```python
from build123d import *

# Parameters (mm, degrees)
F1_DEPTH = 6.35
F2_W     = 6.35
F2_H     = 55.88
F3_DEPTH = 33.64992
F4_SIZE  = 27.94
F5_R     = 10.64163
F6_DEPTH = 38.101


with BuildPart() as f1:
    # F0 (on Top) → F1 (new body)
    with BuildSketch(Plane.XY):
        Polygon((19.05, 27.94), (0, 27.94), (-19.05, 27.94), (-19.05, 0), (-19.05, -27.94), (0, -27.94), (19.05, -27.94), (19.05, 0), align=None)
    extrude(amount=F1_DEPTH)

    # F2 (on face) → F3 (join)
    with BuildSketch(Plane.XY.offset(6.35)):
        with Locations((-15.875, 0)):
            Rectangle(F2_W, F2_H)
        with Locations((15.875, 0)):
            Rectangle(F2_W, F2_H)
    extrude(amount=F3_DEPTH)

    # F4
    f4_edges = [f1.edges().sort_by_distance(p)[0] for p in [
        (15.875, -27.94, 39.99992),
        (-15.875, -27.94, 39.99992),
    ]]
    chamfer(f4_edges, length=F4_SIZE)

    # F5 (on face) → F6 (cut, through all)
    with BuildSketch(Plane.YZ.offset(19.05)):
        with Locations((13.47094, 19.69512)):
            Circle(F5_R)
    extrude(amount=-F6_DEPTH, mode=Mode.SUBTRACT)


solid = f1.part
```
Build history of the part. All positions in model axes, mm. A direction names the side the tool comes from. Give positions to 0.01 mm unless a question says otherwise; leave off trailing zeros. Loops run counter-clockwise (first coordinate to the right, second up) from the corner with the lowest first, then second, coordinate; pieces in that order, holes last.
Item 1: Slice it at B-B, the plane y = 1.5. List the corners of the cut face in (x, z), and give its area (3 significant figures).
Answers follow:
outline: (-19.05, 0) - (19.05, 0) - (19.05, 40) - (12.7, 40) - (12.7, 6.35) - (-12.7, 6.35) - (-12.7, 40) - (-19.05, 40) - close
area: 669 mm2
Item 2: Which spindle directions (+Z, -Z, +X, -X, +Y, -Y) get a long thin tool onto all of the face, cutting with end or side? Do faces 4 (the face through (-13, 27.94, 15)), 5 (the face through (12.7, 0, 23)). Say none if no direction does.
Answers follow:
face 4: +Z, -Z, +X, -X, +Y
face 5: +Z, +Y, -Y
Item 3: Flat gauge pins, fed straight in: pin 1 (1.5 mm diameter, centred on x = -2, y = 3, fed in from +Z); pin 2 (6 mm diameter, centred on x = 10.5, y = -12, fed in from +Z); pin 3 (13 mm diameter, centred on y = 13.47, z = 19.7, fed in from -X); pin 4 (3 mm diameter, centred on x = 14, z = 31, fed in from -Y). Where does each tip first touch, or does it go through?
Answers follow:
pin 1: stops at z = 6.35
pin 2: stops at z = 30.04
pin 3: passes through
pin 4: stops at y = -10.5
Item 4: Slice it at A-A, the plane z = 35. List the corners of the cut face in (x, y).
Answers follow:
outline: (-19.05, -5) - (-12.7, -5) - (-12.7, 27.94) - (-19.05, 27.94) - close; (12.7, -5) - (19.05, -5) - (19.05, 27.94) - (12.7, 27.94) - close
Item 5: Slice it at C-C, the plane z = 24.5. List the corners of the cut face in (x, y).
Answers follow:
outline: (-19.05, -15.5) - (-12.7, -15.5) - (-12.7, 3.98) - (-19.05, 3.98) - close; (-19.05, 22.97) - (-12.7, 22.97) - (-12.7, 27.94) - (-19.05, 27.94) - close; (12.7, -15.5) - (19.05, -15.5) - (19.05, 3.98) - (12.7, 3.98) - close; (12.7, 22.97) - (19.05, 22.97) - (19.05, 27.94) - (12.7, 27.94) - close
Item 6: Slice it at D-D, the plane y = 18.5. List the corners of the cut face in (x, z).
Answers follow:
outline: (-19.05, 0) - (19.05, 0) - (19.05, 10.32) - (12.7, 10.32) - (12.7, 6.35) - (-12.7, 6.35) - (-12.7, 10.32) - (-19.05, 10.32) - close; (-19.05, 29.07) - (-12.7, 29.07) - (-12.7, 40) - (-19.05, 40) - close; (12.7, 29.07) - (19.05, 29.07) - (19.05, 40) - (12.7, 40) - close
Item 7: Pull direction X, two halves, no side cores. Call faces 1 (the face through (16, 14, 40)), 2 (the face through (-12.7, 0, 23)), 3 (the face through (-19.05, 0, 15)): released by +X, released by -X, zero draft, split by the parting line, or undercut.
Answers follow:
face 1: zero draft
face 2: undercut
face 3: released by -X
Item 8: Drill centre lines: line 1 (X direction, y = 0.5, z = 17); line 2 (Z direction, x = 0.5, y = -10.5); line 3 (Y direction, x = 15.5, z = 21.5). Where is each one in solid material? Low to high.
Answers follow:
line 1: x = -19.05 to -12.7, 12.7 to 19.05
line 2: z = 0 to 6.35
line 3: y = -18.5 to 2.98, 23.96 to 27.94
